Could you check a few things on this drawing? It's one solid part, dimensions in mm from its lowest x, y, z. A direction names the side the tool comes from. Give positions to 0.01 mm unless a question says otherwise; leave off trailing zeros. Loops run counter-clockwise (first coordinate to the right, second up) from the corner with the lowest first, then second, coordinate; pieces in that order, holes last. Notation, with made-up numbers: (59.5, 86.5) - (115.5, 86.5) arc R36 ccw to (115.5, 125.5) - close; hole circle Ø10 at (-16, 23). An arc over 180 degrees is marked (long way). Write item = value, one per line.
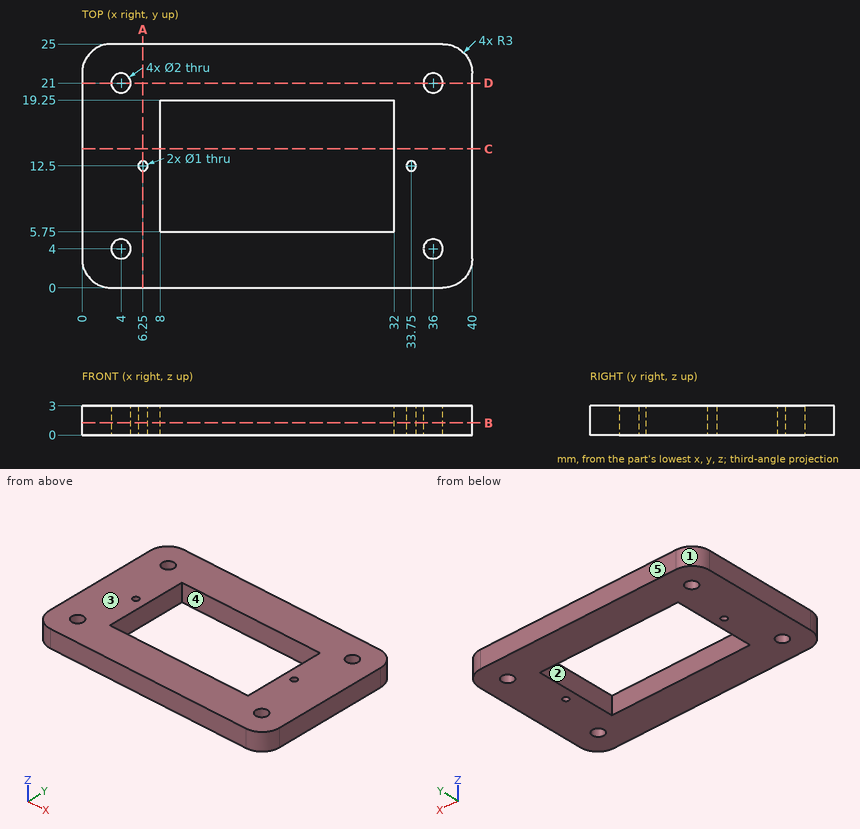
Q1. For pin 1 (2.5 mm diameter, centred on x = 36, y = 21, fed in from +Z); pin 2 (1.8 mm diameter, centred on x = 4, y = 21, fed in from -Z), each with a flat end and sliding along its axis, tell me the tip position at first contact or that it passes through.
Output:
pin_1 = 3
pin_2 = through
Q2. Imagine slicing it at B-B, the plane z = 1.25. Write out the boundary of the cut face in (x, y).
Output:
outline = (0, 3) arc R3 ccw to (3, 0) - (37, 0) arc R3 ccw to (40, 3) - (40, 22) arc R3 ccw to (37, 25) - (3, 25) arc R3 ccw to (0, 22) - close; hole circle Ø2 at (4, 4); hole circle Ø2 at (4, 21); hole circle Ø1 at (6.25, 12.5); hole (8, 5.75) - (32, 5.75) - (32, 19.25) - (8, 19.25) - close; hole circle Ø1 at (33.75, 12.5); hole circle Ø2 at (36, 4); hole circle Ø2 at (36, 21)
Q3. Imagine slicing it at D-D, the plane y = 21. Write out the boundary of the cut face in (x, z).
Output:
outline = (0, 0) - (3, 0) - (3, 3) - (0, 3) - close; (5, 0) - (35, 0) - (35, 3) - (5, 3) - close; (37, 0) - (40, 0) - (40, 3) - (37, 3) - close
Q4. Imagine slicing it at C-C, the plane y = 14.25. Write out the boundary of the cut face in (x, z).
Output:
outline = (0, 0) - (8, 0) - (8, 3) - (0, 3) - close; (32, 0) - (40, 0) - (40, 3) - (32, 3) - close
Q5. We'd pull the mould along X, two halves only. Please class the marked faces 1, 2 and 3: released by +X, released by -X, zero draft, split by the parting line, or undercut.
Output:
face_1 = released by -X
face_2 = undercut
face_3 = zero draft
Q6. Imagine slicing it at A-A, the plane x = 6.25. Write out the boundary of the cut face in (y, z).
Output:
outline = (0, 0) - (12, 0) - (12, 3) - (0, 3) - close; (13, 0) - (25, 0) - (25, 3) - (13, 3) - close
Q7. Which directions (+Z, -Z, +X, -X, +Y, -Y) give clear straight access to the entire face, cutting with the end or side of a thin tool? Please do the marked faces 4 and 5.
Output:
face_4 = +Z, -Z
face_5 = +Z, -Z, +X, -X, +Y
Q8. I need wall thicknesses on L1, parallel to Y at x = 36, z = 1.1; L2, parallel to X at y = 14, z = 2.45; L3, parallel to Y at x = 10, z = 1.85. Which ranges of each line are inside material? Lowest first, please.
Output:
L1 = 0 to 3, 5 to 20, 22 to 25
L2 = 0 to 8, 32 to 40
L3 = 0 to 5.75, 19.25 to 25
